Part print with two shaded views. Sizes in mm from the minimum x, y, z corner. Give positions to 0.01 mm unless a question says otherwise; leave off trailing zeros. Write each loop counter-clockwise with the first axis right and the second up, starting at its lowest first coordinate (ties: lowest second). Pieces come first, ordered by that corner, then holes. Notation, with made-up numbers: M 87.25,-37 L 110.25,-37 A27 ccw 110.25,-8 Z; hole C -14.75,8.25 d2. An arc over 180 degrees is marked long. Return JSON: item names as keys, results as strings. Group by question number.
Q1. Band-saw the part on B-B, the plane x = 4.25. Give the cut face in (y, z).
Q2. Band-saw the part on A-A, the plane z = 14.5. Give the cut face in (x, y), then the cut area to 3 significant figures.
Q3. Wall check: probe 1 along Y at (x, z) = (1.75, 14.5); probe 2 along Z at (x, y) = (2, 13.5); probe 3 along Y at (x, z) = (1.5, 40.5). Give the ranges that are in metal, low to high.
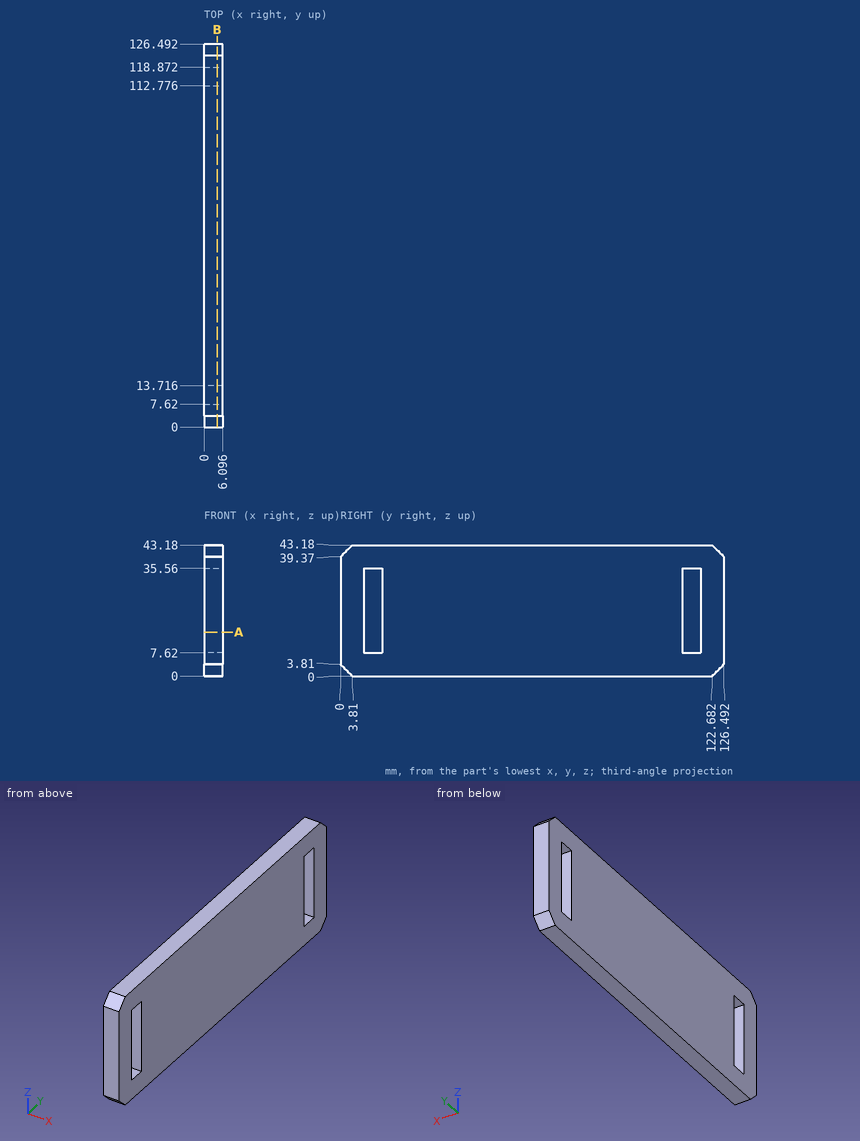
From the geometry:
{
 "1": {"outline": "M 0,3.81 L 3.81,0 L 122.68,0 L 126.49,3.81 L 126.49,39.37 L 122.68,43.18 L 3.81,43.18 L 0,39.37 Z; hole M 7.62,7.62 L 13.72,7.62 L 13.72,35.56 L 7.62,35.56 Z; hole M 112.78,7.62 L 118.87,7.62 L 118.87,35.56 L 112.78,35.56 Z"},
 "2": {"outline": "M 0,0 L 6.1,0 L 6.1,7.62 L 0,7.62 Z; M 0,13.72 L 6.1,13.72 L 6.1,112.78 L 0,112.78 Z; M 0,118.87 L 6.1,118.87 L 6.1,126.49 L 0,126.49 Z", "area": "697 mm^2"},
 "3": {"probe 1": "y = 0 to 7.62, 13.72 to 112.78, 118.87 to 126.49", "probe 2": "z = 0 to 7.62, 35.56 to 43.18", "probe 3": "y = 1.13 to 125.36"}
}
